```python
from build123d import *

# Parameters (mm, degrees)
SKETCH12_W                   = 10.16
SKETCH12_H                   = 228.6
BASE_FLANGE1_DEPTH           = 1.2
EDGE_FLANGE1_STRIP_W         = 6.784000096
EDGE_FLANGE1_STRIP_H         = 1.2
EDGE_FLANGE1_STRIP_CUT_DEPTH = 228.6
EDGE_FLANGE1_DEPTH           = 228.6
EDGE_FLANGE2_STRIP_W         = 6.784000096
EDGE_FLANGE2_STRIP_H         = 1.2
EDGE_FLANGE2_STRIP_CUT_DEPTH = 228.6
EDGE_FLANGE2_DEPTH           = 228.6
EDGE_FLANGE3_STRIP_W         = 6.784000096
EDGE_FLANGE3_STRIP_H         = 1.2
EDGE_FLANGE3_STRIP_CUT_DEPTH = 228.6
EDGE_FLANGE3_DEPTH           = 228.6
F_1_4_0_25_DIAMETER_HOLE1_D  = 6.35
CUT_EXTRUDE1_DEPTH           = 116.034681727
CUT_EXTRUDE1_DEPTH_BACK      = 116.034681727
SKETCH30_R                   = 3.175
CLOSED_START                 = -114.3
CLOSED_CORNER1_OUTLINE_W     = 0.127
CLOSED_CORNER1_OUTLINE_H     = 1.2
CLOSED_CORNER1_DEPTH         = 228.6
CLOSED_CORNER1_2_OUTLINE_W   = 1.2
CLOSED_CORNER1_2_OUTLINE_H   = 6.35
CLOSED_CORNER1_2_DEPTH       = 228.6
FILLET1_R                    = 2.54


# Read off the part's stored shape, not the designer's step: Closed Corner1
# Sheet-metal steps are written as plain solids
with BuildPart() as part:
    # Sketch12 → Base-Flange1 (new body)
    with BuildSketch(Plane.XY):
        Rectangle(SKETCH12_W, SKETCH12_H)
    extrude(amount=-BASE_FLANGE1_DEPTH)

    # Edge-Flange1 strip (across the edge) → Edge-Flange1 strip cut (cut)
    with BuildSketch(Plane(origin=(-5.08, 114.3, 0), x_dir=(1, 0, 0), z_dir=(0, -1, 0))):
        with Locations((-1.2, -0.6)):
            Rectangle(EDGE_FLANGE1_STRIP_W, EDGE_FLANGE1_STRIP_H)
    extrude(amount=EDGE_FLANGE1_STRIP_CUT_DEPTH, mode=Mode.SUBTRACT)

    # Edge-Flange1 section (across the edge) → Edge-Flange1 (add)
    with BuildSketch(Plane(origin=(-5.08, 114.3, 0), x_dir=(1, 0, 0), z_dir=(0, -1, 0))):
        with BuildLine():
            Line((0, 0.992000048), (0, 10.16))
            Line((0, 10.16), (1.2, 10.16))
            Line((1.2, 10.16), (1.2, 0.992000048))
            ThreePointArc((1.2, 0.992000048), (1.490550087, 0.290550087), (2.192000048, 0))
            Line((2.192000048, 0), (2.192000048, -1.2))
            ThreePointArc((2.192000048, -1.2), (0.64202195, -0.55797805), (0, 0.992000048))
        make_face()
    extrude(amount=EDGE_FLANGE1_DEPTH)

    # Edge-Flange2 strip (across the edge) → Edge-Flange2 strip cut (cut)
    with BuildSketch(Plane(origin=(-3.88, 114.3, 10.16), x_dir=(0, 0, -1), z_dir=(0, -1, 0))):
        with Locations((-1.2, -0.6)):
            Rectangle(EDGE_FLANGE2_STRIP_W, EDGE_FLANGE2_STRIP_H)
    extrude(amount=EDGE_FLANGE2_STRIP_CUT_DEPTH, mode=Mode.SUBTRACT)

    # Edge-Flange2 section (across the edge) → Edge-Flange2 (add)
    with BuildSketch(Plane(origin=(-3.88, 114.3, 10.16), x_dir=(0, 0, -1), z_dir=(0, -1, 0))):
        with BuildLine():
            Line((0, 0.992000048), (0, 8.96))
            Line((0, 8.96), (1.2, 8.96))
            Line((1.2, 8.96), (1.2, 0.992000048))
            ThreePointArc((1.2, 0.992000048), (1.490550087, 0.290550087), (2.192000048, 0))
            Line((2.192000048, 0), (2.192000048, -1.2))
            ThreePointArc((2.192000048, -1.2), (0.64202195, -0.55797805), (0, 0.992000048))
        make_face()
    extrude(amount=EDGE_FLANGE2_DEPTH)

    # Edge-Flange3 strip (across the edge) → Edge-Flange3 strip cut (cut)
    with BuildSketch(Plane(origin=(5.08, 114.3, 8.96), x_dir=(-1, 0, 0), z_dir=(0, -1, 0))):
        with Locations((-2.4, -0.6)):
            Rectangle(EDGE_FLANGE3_STRIP_W, EDGE_FLANGE3_STRIP_H)
    extrude(amount=EDGE_FLANGE3_STRIP_CUT_DEPTH, mode=Mode.SUBTRACT)

    # Edge-Flange3 section (across the edge) → Edge-Flange3 (add)
    with BuildSketch(Plane(origin=(5.08, 114.3, 8.96), x_dir=(-1, 0, 0), z_dir=(0, -1, 0))):
        with BuildLine():
            Line((-1.2, 0.992000048), (-1.2, 3.81))
            Line((-1.2, 3.81), (0, 3.81))
            Line((0, 3.81), (0, 0.992000048))
            ThreePointArc((0, 0.992000048), (0.290550087, 0.290550087), (0.992000048, 0))
            Line((0.992000048, 0), (0.992000048, -1.2))
            ThreePointArc((0.992000048, -1.2), (-0.55797805, -0.55797805), (-1.2, 0.992000048))
        make_face()
    extrude(amount=EDGE_FLANGE3_DEPTH)

    # 1/4 (0.25) Diameter Hole1 (through all)
    with Locations(Plane.XY.offset(10.16)):
        with Locations((0.6, 0)):
            Hole(F_1_4_0_25_DIAMETER_HOLE1_D / 2)

    # Sketch30 → Cut-Extrude1 (cut, two sides: drawn at the far end of the back side and taken through both)
    with BuildSketch(Plane.XY.offset(10.16).offset(-CUT_EXTRUDE1_DEPTH_BACK)):
        with Locations((0.6, -109.22)):
            Circle(SKETCH30_R)
        with Locations((0.6, 109.22)):
            Circle(SKETCH30_R)
    extrude(amount=CUT_EXTRUDE1_DEPTH + CUT_EXTRUDE1_DEPTH_BACK, mode=Mode.SUBTRACT)

    # Closed Corner1 outline → Closed Corner1 (cut)
    with BuildSketch(Plane(origin=(0, 0, 0), x_dir=(1, 0, 0), z_dir=(0, 1, 0)).offset(CLOSED_START)):
        with Locations((5.0165, 0.6)):
            Rectangle(CLOSED_CORNER1_OUTLINE_W, CLOSED_CORNER1_OUTLINE_H)
    extrude(amount=CLOSED_CORNER1_DEPTH, mode=Mode.SUBTRACT)

    # Closed Corner1 2 outline → Closed Corner1 2 (add)
    with BuildSketch(Plane(origin=(0, 0, 0), x_dir=(1, 0, 0), z_dir=(0, 1, 0)).offset(CLOSED_START)):
        with Locations((5.68, -1.975)):
            Rectangle(CLOSED_CORNER1_2_OUTLINE_W, CLOSED_CORNER1_2_OUTLINE_H)
    extrude(amount=CLOSED_CORNER1_2_DEPTH)

    # Fillet1
    # the kernel refuses this fillet: 2.54 mm, written as the material it takes off along each edge
    with BuildSketch(Plane(origin=(6.28, -119.694441584, -1.2), x_dir=(0, 0, 1), z_dir=(0, 1, 0))) as fillet1_piece_1:
        with BuildLine():
            CenterArc((2.157776633, -2.54), FILLET1_R, 90, 58.159322109)
            Line((0, -1.2), (-0.043155533, -1.1732))
            ThreePointArc((-0.043155533, -1.1732), (-0.0508, -0.6), (-0.0508, 0))
            Line((-0.0508, 0), (0, 0.0508))
            Line((0, 0.0508), (2.157776633, 0.0508))
            Line((2.157776633, 0.0508), (2.157776633, 0))
        make_face()
    extrude(amount=239.388883167, mode=Mode.SUBTRACT)


solid = part.part
```
Design review of the part built by this model. Coordinates are the model's own, in mm. A direction names the side the tool comes from. Coordinates: 2 decimals unless noted, no trailing zeros. Order: outer loops, then holes, each group sorted by start corner. A loop starts at its lowest first (then second) coordinate and runs counter-clockwise, first axis right, second up.
1) Clearance check with flat-ended pins moving along their axes: pin 1 (1 mm diameter, centred on y = -51, z = -0.5, fed in from +X); pin 2 (5.5 mm diameter, centred on x = 0.6, y = -109.22, fed in from +Z); pin 3 (5 mm diameter, centred on x = -0.5, z = 1.5, fed in from -Y). State where each tip first meets the part, or that it passes through.
2) Take a section at D-D, the plane y = -53. Give the boundary of the cut face in (x, z).
3) Take a section at B-B, the plane y = -109.22. Give the boundary of the cut face in (x, z) (3 decimals), and give its area (3 significant figures).
4) Take a section at A-A, the plane z = 3.5. Give the boundary of the cut face in (x, y), and give its area (3 significant figures).
5) Take a section at C-C, the plane x = 0.6. State how many separate pieces and enclosed holes the cut face has, and give its area (3 significant figures).
6) For faces 4 (the cylindrical face through (-2.43, 0.95, 9.55)), 5 (the flat face through (4, 2, 0)), list the 3-axis set-ups (+Z, -Z, +X, -X, +Y, -Y) from which the entire face can be reached by the end or side of a thin tool; tool diameter is ignored.
7) Mouldability with a two-part tool opening along Y and no side actions: class faces 1 (the flat face through (6, 114.3, 4)), 2 (the flat face through (4, 2, -1.2)), 3 (the cylindrical face through (-2.43, 0.95, -0.61)) as +Y half, -Y half, draft (parallel to the pull), parting line (faces both ways), or undercut.
8) Wall thickness on line 1 along Y through (x, z) = (0.6, 9.75) (3 decimals); line 2 along X through (y, z) = (-78, 8.25); line 3 along X through (y, z) = (68.5, 5.75): over which ranges is each line inside the solid? List them lowest first.
Returned:
1. pin 1: stops at x = 6.09
1. pin 2: passes through
1. pin 3: stops at y = -114.3
2. outline: (-5.08, 0.99) arc R2.19 ccw to (-2.89, -1.2) - (4.95, -1.2) - (4.95, 0) - (-2.89, 0) arc R0.99 cw to (-3.88, 0.99) - (-3.88, 7.97) arc R0.99 cw to (-2.89, 8.96) - (4.09, 8.96) arc R0.99 cw to (5.08, 7.97) - (5.08, -1.2) arc R2.54 ccw to (6.28, 0.96) - (6.28, 7.97) arc R2.19 ccw to (4.09, 10.16) - (-2.89, 10.16) arc R2.19 ccw to (-5.08, 7.97) - close
3. outline: (-5.08, 0.992) arc R2.192 ccw to (-2.888, -1.2) - (-2.575, -1.2) - (-2.575, 0) - (-2.888, 0) arc R0.992 cw to (-3.88, 0.992) - (-3.88, 7.968) arc R0.992 cw to (-2.888, 8.96) - (-2.575, 8.96) - (-2.575, 10.16) - (-2.888, 10.16) arc R2.192 ccw to (-5.08, 7.968) - close; (3.775, -1.2) - (4.953, -1.2) - (4.953, 0) - (3.775, 0) - close; (3.775, 8.96) - (4.088, 8.96) arc R0.992 cw to (5.08, 7.968) - (5.08, -1.2) arc R2.54 ccw to (6.28, 0.958) - (6.28, 7.968) arc R2.192 ccw to (4.088, 10.16) - (3.775, 10.16) - close
3. area: 30.2 mm2
4. outline: (-5.08, -114.3) - (-3.88, -114.3) - (-3.88, 114.3) - (-5.08, 114.3) - close; (5.08, -114.3) - (6.28, -114.3) - (6.28, 114.3) - (5.08, 114.3) - close
4. area: 549 mm2
5. separate pieces: 8
5. enclosed holes: 0
5. area: 503 mm2
6. face 4: +Z, -Z
6. face 5: +Y, -Y
7. face 1: +Y half
7. face 2: draft
7. face 3: undercut
8. line 1: y = -114.3 to -112.395, -106.045 to -3.175, 3.175 to 106.045, 112.395 to 114.3
8. line 2: x = -5.06 to -3.84, 5.04 to 6.26
8. line 3: x = -5.08 to -3.88, 5.08 to 6.28
